For this review, take the finished solid that the model builds, in its own axes (mm). Face numbers are marked on the shaded views. A direction names the side the tool comes from. Round coordinates to 2 decimals unless told otherwise and drop trailing zeros. Order: outer loops, then holes, each group sorted by start corner. A loop starts at its lowest first (then second) coordinate and runs counter-clockwise, first axis right, second up. Notation, with made-up numbers: M 60.25,72 L 80.25,72 A35 ccw 80.25,105 Z; hole C 56,44.5 d9. An arc over 180 degrees is marked long. Put each result on its own line as item: value.
from build123d import *

# Parameters (mm, degrees)
SKETCH1_R                      = 4.7625
SKETCH1_R_2                    = 1.5875
BOSS_EXTRUDE1_DEPTH            = 5
BOSS_EXTRUDE2_START            = -5
SKETCH1_3_R                    = 4.7625
SKETCH1_3_R_2                  = 2
BOSS_EXTRUDE2_DEPTH            = 5
SKETCH3_W                      = 1.25
SKETCH3_H                      = 4.7625
M3X0_5_TAPPED_HOLE1_AT_2_COUNT = 2
M3X0_5_TAPPED_HOLE1_AT_2_PITCH = 5.356303923
CHAMFER1_SIZE                  = 0.1


with BuildPart() as part:
    # Sketch1 → Boss-Extrude1 (new body)
    with BuildSketch(Plane.XY):
        Circle(SKETCH1_R)
        Circle(SKETCH1_R_2, mode=Mode.SUBTRACT)
    extrude(amount=BOSS_EXTRUDE1_DEPTH)

    # Sketch1<3> → Boss-Extrude2 (add)
    with BuildSketch(Plane.XY.offset(BOSS_EXTRUDE2_START)):
        Circle(SKETCH1_3_R)
        Circle(SKETCH1_3_R_2, mode=Mode.SUBTRACT)
    extrude(amount=BOSS_EXTRUDE2_DEPTH)

    # Sketch3 → M3x0.5 Tapped Hole1 (revolve, cut)
    with BuildSketch(Plane(origin=(0, 0, 2.591545057), x_dir=(0, 0, -1), z_dir=(1, 0, 0))):
        with Locations((0.625, 2.38125)):
            Rectangle(SKETCH3_W, SKETCH3_H)
    m3x0_5_tapped_hole1 = revolve(axis=Axis((0, -6.35, 2.591545057), (0, 1, 0)), mode=Mode.SUBTRACT)

    # M3x0.5 Tapped Hole1 at 2: M3x0.5 Tapped Hole1 ×2
    with Locations(*[(0, 0, -i * M3X0_5_TAPPED_HOLE1_AT_2_PITCH) for i in range(1, M3X0_5_TAPPED_HOLE1_AT_2_COUNT)]):
        add(m3x0_5_tapped_hole1, mode=Mode.SUBTRACT)

    # Chamfer1
    chamfer1_edges = [part.edges().sort_by_distance(p)[0] for p in [
        (-4.7625, 0, -5),
        (-2, 0, -5),
        (-4.7625, 0, 5),
        (-1.5875, 0, 5),
    ]]
    chamfer(chamfer1_edges, length=CHAMFER1_SIZE)


solid = part.part
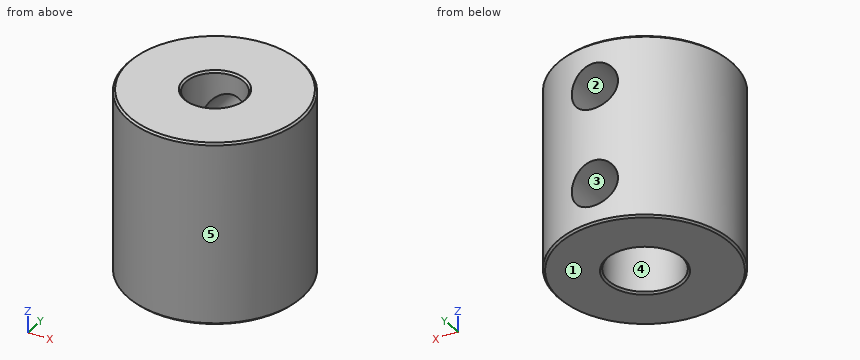
(1) Add section C-C on z = -0.25. Give the boundary of the cut face in (x, y) (1 decimal).
A:
outline: C 0,0 d9.5; hole C 0,0 d4
(2) To check wall thickness, follow L1, parallel to Z at x = 0, y = 2.3; L2, parallel to Z at x = 1.75, y = 0; L3, parallel to Y at x = -1.25, z = -1. State the ranges of each line that lie inside material, in increasing order.
A:
L1: z = -5 to -4.01, -1.51 to 1.34, 3.84 to 5
L2: z = 0 to 5
L3: y = -4.6 to -1.56, 1.56 to 4.6
(3) Insertion check: pin 1 Ø1.5 at (x, z) = (0, 2.59) entering from +Y; pin 2 Ø3 at (x, y) = (0, 0) entering from -Z; pin 3 Ø3 at (x, z) = (3, -1) entering from -Y; pin 4 Ø5 at (x, z) = (-3.5, 0.5) entering from +Y. Each pin has a flat end and moves straight along its axis. Give the tip position at first contact, or say it passes through.
A:
pin 1: stops at y = -1.4
pin 2: passes through
pin 3: stops at y = -4.52
pin 4: stops at y = 4.66
(4) Add section A-A on x = 0. Give the boundary of the cut face in (y, z), then the cut area to 3 significant figures.
A:
outline: M -4.76,-4.9 L -4.66,-5 L -2.1,-5 L -2,-4.9 L -2,0 L -1.59,0 L -1.59,4.9 L -1.69,5 L -4.66,5 L -4.76,4.9 Z; M 1.59,0 L 2,0 L 2,-1.51 L 4.76,-1.51 L 4.76,1.34 L 1.59,1.34 Z; M 1.59,3.84 L 4.76,3.84 L 4.76,4.9 L 4.66,5 L 1.69,5 L 1.59,4.9 Z; M 2,-4.9 L 2.1,-5 L 4.66,-5 L 4.76,-4.9 L 4.76,-4.01 L 2,-4.01 Z
area: 44.5 mm2
(5) Add section D-D on z = -2. Give the boundary of the cut face in (x, y) (1 decimal).
A:
outline: M -1,1.7 L -1,4.7 A4.8 ccw long 1,4.7 L 1,1.7 A2 cw long Z
(6) Draft analysis for pull direction Y (two halves, no side actions). For the marked faces 3, 4 and 5, state which applies: released by +Y, released by -Y, zero draft, split by the parting line, or undercut.
A:
face 3: zero draft
face 4: undercut
face 5: split by the parting line
(7) For the marked faces 1 and 2, list the 3-axis set-ups (+Z, -Z, +X, -X, +Y, -Y) from which the entire face can be reached by the end or side of a thin tool; tool diameter is ignored.
A:
face 1: -Z, +X, -X, +Y, -Y
face 2: +Y
(8) Add section B-B on y = 0. Give the boundary of the cut face in (x, z), then the cut area to 3 significant figures.
A:
outline: M -4.76,-4.9 L -4.66,-5 L -2.1,-5 L -2,-4.9 L -2,0 L -1.59,0 L -1.59,4.9 L -1.69,5 L -4.66,5 L -4.76,4.9 Z; M 1.59,0 L 2,0 L 2,-4.9 L 2.1,-5 L 4.66,-5 L 4.76,-4.9 L 4.76,4.9 L 4.66,5 L 1.69,5 L 1.59,4.9 Z
area: 59.3 mm2
